Answer from the drawing. Dimensions are ordinates in mm from the lowest x, y and z of the part. A direction names the side the tool comes from. Coordinates: 2 decimals unless noted, no trailing zeros. Order: outer loops, then holes, each group sorted by start corner. A loop starts at its lowest first (then second) coordinate and runs counter-clockwise, first axis right, second up. Notation, with made-up numbers: M 87.25,6 L 107.25,6 A21 ccw 107.25,18 Z; hole C 30,43.5 d3. An arc over 180 degrees is marked long. Write each question's results on one line, items separated by ' | '.
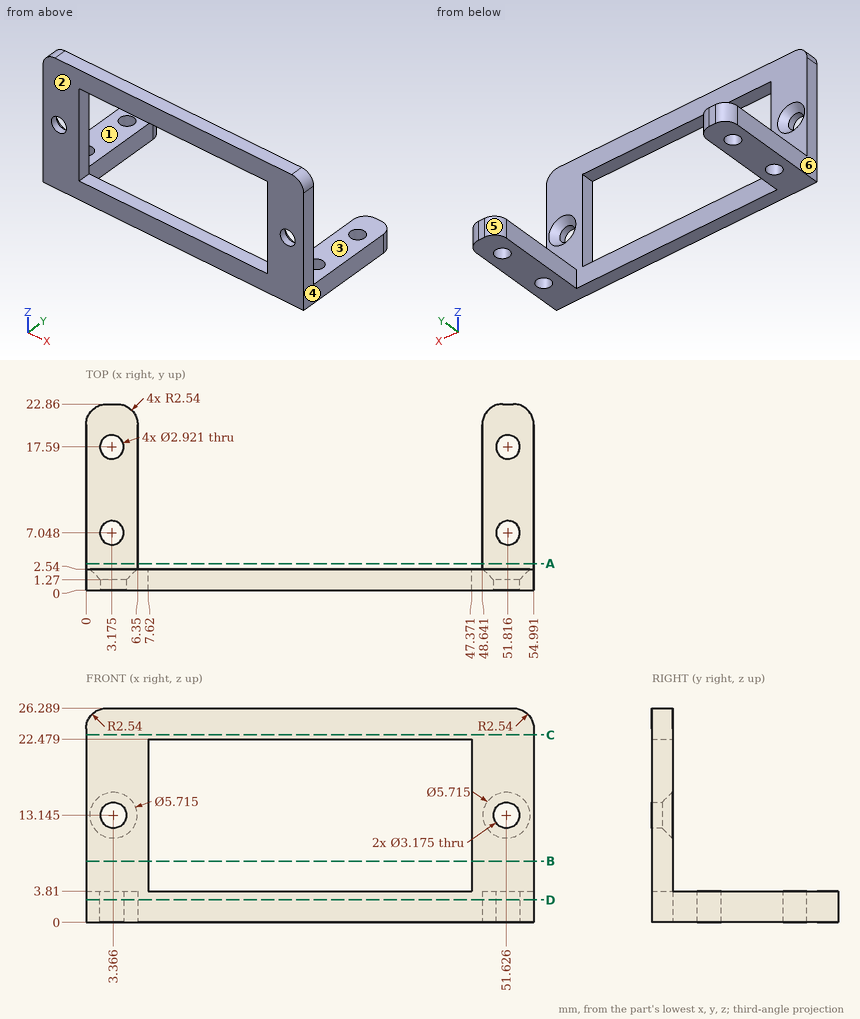
(1) The part is cut by section D-D, the plane z = 2.75. Count the separate pieces of the cut face and the enclosed holes in it.
Conclusion:
separate pieces: 1 | enclosed holes: 4
(2) Straight lines are drawn through the part: line 1 (X direction, y = 1.5, z = 8); line 2 (X direction, y = 20.25, z = 2.75); line 3 (Z direction, x = 13.5, y = 2.5). For each, find the intervals that lie inside material, in ascending order.
Conclusion:
line 1: 0 to 7.62, 47.37 to 54.99 | line 2: 0 to 6.35, 48.64 to 54.99 | line 3: 0 to 3.81, 22.48 to 26.29
(3) For the marked faces 1 and 2, determine the directions among +Z, -Z, +X, -X, +Y, -Y from which every point of the face is accessible in a straight line to the end or side of a thin tool.
Conclusion:
face 1: +Z, +X, -X, +Y | face 2: +Z, -Z, +X, -X, -Y
(4) Given pin 1 (12 mm diameter, centred on x = 13, z = 23, fed in from +Y); pin 2 (3 mm diameter, centred on x = 3.5, y = 9, fed in from +Z), each flat-ended and moving along its own axis, determine where each tip first touches the part or whether it passes through.
Conclusion:
pin 1: y = 2.54 | pin 2: z = 3.81
(5) The part is cut by section A-A, the plane y = 3.25. Write down the section's boundary in (x, z).
Conclusion:
outline: M 0,0 L 6.35,0 L 6.35,3.81 L 0,3.81 Z; M 48.64,0 L 54.99,0 L 54.99,3.81 L 48.64,3.81 Z
(6) The mould has two halves that part along X. Classify the marked faces 3, 4, 5 and 6: pulls with the +X half, pulls with the -X half, needs draft (parallel to the pull), parting line crosses it, or undercut.
Conclusion:
face 3: needs draft | face 4: pulls with the +X half | face 5: undercut | face 6: pulls with the -X half
(7) The part is cut by section B-B, the plane z = 7.5. Write down the section's boundary in (x, y).
Conclusion:
outline: M 0,0 L 7.62,0 L 7.62,2.54 L 0,2.54 Z; M 47.37,0 L 54.99,0 L 54.99,2.54 L 47.37,2.54 Z
(8) The part is cut by section C-C, the plane z = 23. Write down the section's boundary in (x, y).
Conclusion:
outline: M 0,0 L 54.99,0 L 54.99,2.54 L 0,2.54 Z
